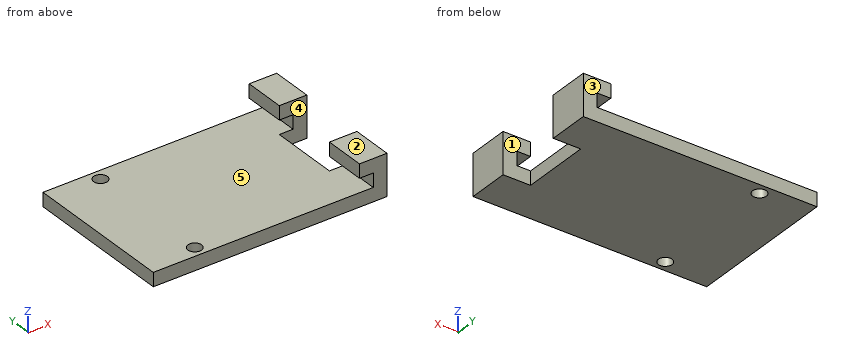
```python
from build123d import *

# Parameters (mm, degrees)
F0_W     = 85
F0_H     = 55
F1_DEPTH = 5
F2_W     = 55
F2_H     = 10
F3_DEPTH = 5
F4_W     = 55
F4_H     = 5
F5_DEPTH = 10
F6_W     = 10
F6_H     = 25
F7_DEPTH = 23.6
F8_R     = 2.5
F9_DEPTH = 25


with BuildPart() as f1:
    # F0 (on Top) → F1 (new body)
    with BuildSketch(Plane.XY):
        with Locations((-0.6882026792, -4.6636614819)):
            Rectangle(F0_W, F0_H)
    extrude(amount=F1_DEPTH)

    # F2 (on face) → F3 (join)
    with BuildSketch(Plane.YZ.offset(41.8117973208)):
        with Locations((-4.6636614819, 5)):
            Rectangle(F2_W, F2_H)
    extrude(amount=-F3_DEPTH)

    # F4 (on face) → F5 (join)
    with BuildSketch(Plane.YZ.offset(41.8117973208)):
        with Locations((-4.6636614819, 12.5)):
            Rectangle(F4_W, F4_H)
    extrude(amount=-F5_DEPTH)

    # F6 (on face) → F7 (cut)
    with BuildSketch(Plane.XY.offset(15)):
        with Locations((36.8117973208, -4.6636614819)):
            Rectangle(F6_W, F6_H)
    extrude(amount=-F7_DEPTH, mode=Mode.SUBTRACT)

    # F8 (on face) → F9 (cut)
    with BuildSketch(Plane.XY.offset(5)):
        with Locations((-25.1882026792, -28.1636614819)):
            Circle(F8_R)
        with Locations((-25.1882026792, 18.8363385181)):
            Circle(F8_R)
    extrude(amount=-F9_DEPTH, mode=Mode.SUBTRACT)


solid = f1.part
```
The listing builds one solid part. Answer for the finished solid, in the listing's coordinates (mm). Face numbers are marked on the shaded views. A direction names the side the tool comes from. Round coordinates to 2 decimals unless told otherwise and drop trailing zeros. Loops run counter-clockwise (first coordinate to the right, second up) from the corner with the lowest first, then second, coordinate; pieces in that order, holes last.
Q1. Which of the six approach directions +Z, -Z, +X, -X, +Y, -Y give full straight-line access (tool end or side, diameter ignored) to the marked faces 1 and 2?
Q2. Section B-B, the plane y = -27 is taken. Determine the outline of the cut face in (x, z).
Q3. For a pull along Y with two mould halves and no side action, classify the marked faces 3, 4 and 5 as released by +Y, released by -Y, zero draft, split by the parting line, or undercut.
Q4. Section C-C, the plane z = 6 is taken. Determine the outline of the cut face in (x, y), then the cut area to 3 significant figures.
Q5. Section A-A, the plane z = 11 is taken. Determine the outline of the cut face in (x, y), then the cut area to 3 significant figures.
Q6. Section D-D, the plane y = 12.5 is taken. Determine the outline of the cut face in (x, z), then the cut area to 3 significant figures.
Q7. Given pin 1 Ø3 at (x, z) = (-8, 7.5) entering from +Y; pin 2 Ø5.5 at (y, z) = (-28.5, 8) entering from -X; pin 3 Ø10 at (x, y) = (-24.5, -7.5) entering from +Z; pin 4 Ø4 at (y, z) = (18, 7.5) entering from -X, each flat-ended and moving along its own axis, determine where each tip first touches the part or whether it passes through.
Q8. Find the intervals of material crossed by line 1 (Z direction, x = -12, y = 9); line 2 (X direction, y = 8.5, z = 7.5), in increasing order.
Completed:
1. face 1: +Z, -Z, +X
1. face 2: +Z, +X, -X, +Y, -Y
2. outline: (-43.19, 0) - (-27.4, 0) - (-27.4, 5) - (-43.19, 5) - close; (-22.98, 0) - (41.81, 0) - (41.81, 15) - (31.81, 15) - (31.81, 10) - (36.81, 10) - (36.81, 5) - (-22.98, 5) - close
3. face 3: released by +Y
3. face 4: undercut
3. face 5: zero draft
4. outline: (36.81, -32.16) - (41.81, -32.16) - (41.81, -17.16) - (36.81, -17.16) - close; (36.81, 7.84) - (41.81, 7.84) - (41.81, 22.84) - (36.81, 22.84) - close
4. area: 150 mm2
5. outline: (31.81, -32.16) - (41.81, -32.16) - (41.81, -17.16) - (31.81, -17.16) - close; (31.81, 7.84) - (41.81, 7.84) - (41.81, 22.84) - (31.81, 22.84) - close
5. area: 300 mm2
6. outline: (-43.19, 0) - (41.81, 0) - (41.81, 15) - (31.81, 15) - (31.81, 10) - (36.81, 10) - (36.81, 5) - (-43.19, 5) - close
6. area: 500 mm2
7. pin 1: passes through
7. pin 2: stops at x = 31.81
7. pin 3: stops at z = 5
7. pin 4: stops at x = 36.81
8. line 1: z = 0 to 5
8. line 2: x = 36.81 to 41.81
